Work out the finished part from the listing and answer in its coordinate system (mm). Face numbers are marked on the shaded views. A direction names the side the tool comes from. Round coordinates to 2 decimals unless told otherwise and drop trailing zeros. Write each loop counter-clockwise with the first axis right and the second up, starting at its lowest first coordinate (ties: lowest second). Pieces come first, ordered by that corner, then holes. Notation, with made-up numbers: M 7,13 L 58,13 A18 ccw 58,39 Z; hole C 4,82 d4. An arc over 180 degrees is marked long. Answer in a Markdown table with one row per item.
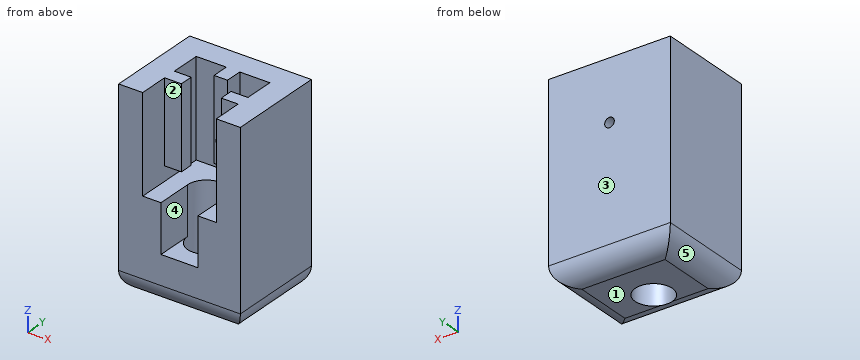
```python
from build123d import *

# Parameters (mm, degrees)
RESSALTO_EXTRUS_O1_DEPTH   = 20
ESBO_O2_W                  = 25.3
ESBO_O2_H                  = 20.3
ESBO_O2_R                  = 3.85
RESSALTO_EXTRUS_O2_DEPTH   = 20
CORTE_EXTRUS_O1_DEPTH      = 10
ESBO_O3_W                  = 3.5
ESBO_O3_H                  = 2.8
ESBO_O3_W_2                = 2.8
ESBO_O3_H_2                = 3.5
RESSALTO_EXTRUS_O3_DEPTH   = 17
CORTE_EXTRUS_O2_DEPTH      = 29.180001774
CORTE_EXTRUS_O2_DEPTH_BACK = 29.180001774
ESBO_O4_R                  = 1
FILETE1_R                  = 4


with BuildPart() as part:
    # Esboço1 → Ressalto-extrusão1 (new body)
    with BuildSketch(Plane.XY):
        Polygon((-7.65, 0), (-12.65, 0), (-12.65, 20.3), (12.65, 20.3), (12.65, 0), (7.65, 0), (7.65, 15.3), (-7.65, 15.3), align=None)
    extrude(amount=RESSALTO_EXTRUS_O1_DEPTH)

    # Esboço2 → Ressalto-extrusão2 (add)
    with BuildSketch(Plane(origin=(0, 0, 0), x_dir=(-1, 0, 0), z_dir=(0, 0, -1))):
        with Locations((0, 10.15)):
            Rectangle(ESBO_O2_W, ESBO_O2_H)
        with Locations((0, 7.65)):
            Circle(ESBO_O2_R, mode=Mode.SUBTRACT)
    extrude(amount=RESSALTO_EXTRUS_O2_DEPTH)

    # Esboço2<3> → Corte-extrusão1 (cut)
    with BuildSketch(Plane(origin=(0, 0, 0), x_dir=(-1, 0, 0), z_dir=(0, 0, -1))):
        with BuildLine():
            Line((3.85, 3.8), (2.722361108, 4.927638892))
            ThreePointArc((2.722361108, 4.927638892), (-1.473331215, 4.0930638), (-3.85, 7.65))
            Line((-3.85, 7.65), (-3.85, 0))
            Line((-3.85, 0), (3.85, 0))
            Line((3.85, 0), (3.85, 3.8))
        make_face()
        with BuildLine():
            ThreePointArc((3.85, 7.65), (3.5569362, 6.176668785), (2.722361108, 4.927638892))
            Line((2.722361108, 4.927638892), (3.85, 3.8))
            Line((3.85, 3.8), (3.85, 7.65))
        make_face()
    extrude(amount=CORTE_EXTRUS_O1_DEPTH, mode=Mode.SUBTRACT)

    # Esboço3 → Ressalto-extrusão3 (add)
    with BuildSketch(Plane.XY.offset(20)):
        with Locations((5.9, 7.65)):
            Rectangle(ESBO_O3_W, ESBO_O3_H)
        with Locations((-5.9, 7.65)):
            Rectangle(ESBO_O3_W, ESBO_O3_H)
        with Locations((0, 13.55)):
            Rectangle(ESBO_O3_W_2, ESBO_O3_H_2)
    extrude(amount=-RESSALTO_EXTRUS_O3_DEPTH)

    # Esboço4 → Corte-extrusão2 (cut, two sides: drawn at the far end of the back side and taken through both)
    with BuildSketch(Plane.XZ.offset(-15.3).offset(-CORTE_EXTRUS_O2_DEPTH_BACK)):
        with Locations(Location((0, 7.5, 0), (0, 0, 270))):
            Circle(ESBO_O4_R)
    extrude(amount=CORTE_EXTRUS_O2_DEPTH + CORTE_EXTRUS_O2_DEPTH_BACK, mode=Mode.SUBTRACT)

    # Filete1
    # the kernel refuses this fillet: 4 mm, written as the material it takes off along each edge
    with BuildSketch(Plane(origin=(12.65, -10, -20), x_dir=(-1, 0, 0), z_dir=(0, 1, 0))) as filete1_piece_1:
        with BuildLine():
            CenterArc((FILETE1_R, FILETE1_R), FILETE1_R, 180, 90)
            Line((0, FILETE1_R), (0, 0))
            Line((0, 0), (FILETE1_R, 0))
        make_face()
    extrude(amount=40.3, mode=Mode.SUBTRACT)
    with BuildSketch(Plane(origin=(-22.65, 0, -20), x_dir=(0, 0, 1), z_dir=(1, 0, 0)), Plane(origin=(22.65, 20.3, -20), x_dir=(0, 0, 1), z_dir=(-1, 0, 0))) as filete1_piece_2:
        with BuildLine():
            CenterArc((FILETE1_R, -FILETE1_R), FILETE1_R, 90, 90)
            Line((0, -FILETE1_R), (0, 0))
            Line((0, 0), (FILETE1_R, 0))
        make_face()
    extrude(amount=45.3, mode=Mode.SUBTRACT)
    with BuildSketch(Plane(origin=(-12.65, 30.3, -20), x_dir=(0, 0, 1), z_dir=(0, -1, 0))) as filete1_piece_3:
        with BuildLine():
            CenterArc((FILETE1_R, -FILETE1_R), FILETE1_R, 90, 90)
            Line((0, -FILETE1_R), (0, 0))
            Line((0, 0), (FILETE1_R, 0))
        make_face()
    extrude(amount=40.3, mode=Mode.SUBTRACT)


solid = part.part
```
1. The part is cut by section B-B (z = 8). Determine the outline of the cut face in (x, y), plus the area to 3 significant figures.
Calculated:
| item | result |
|---|---|
| outline | M -12.65,0 L -7.65,0 L -7.65,6.25 L -4.15,6.25 L -4.15,9.05 L -7.65,9.05 L -7.65,15.3 L -1.4,15.3 L -1.4,11.8 L -0.87,11.8 L -0.87,20.3 L -12.65,20.3 Z; M 0.87,11.8 L 1.4,11.8 L 1.4,15.3 L 7.65,15.3 L 7.65,9.05 L 4.15,9.05 L 4.15,6.25 L 7.65,6.25 L 7.65,0 L 12.65,0 L 12.65,20.3 L 0.87,20.3 Z |
| area | 294 mm² |
2. A tool of negligible diameter and unlimited length cuts with its end or side. For the marked faces 1 and 2, from which of +Z, -Z, +X, -X, +Y, -Y can it reach the whole face along a straight path? Write none if from no direction.
Calculated:
| item | result |
|---|---|
| face 1 | -Z, +X, -X, +Y, -Y |
| face 2 | +Z, -Y |
3. The part is cut by section A-A (x = 7). Determine the outline of the cut face in (y, z), plus the area to 3 significant figures.
Calculated:
| item | result |
|---|---|
| outline | M 0,-16 A4 ccw 4,-20 L 16.3,-20 A4 ccw 20.3,-16 L 20.3,20 L 15.3,20 L 15.3,0 L 0,0 Z; M 6.25,3 L 9.05,3 L 9.05,20 L 6.25,20 Z |
| area | 547 mm² |
4. The part is cut by section C-C (y = 4.5). Determine the outline of the cut face in (x, z), plus the area to 3 significant figures.
Calculated:
| item | result |
|---|---|
| outline | M -12.65,-16 A4 ccw -8.65,-20 L -2.21,-20 L -2.21,-10 L -3.85,-10 L -3.85,0 L -7.65,0 L -7.65,20 L -12.65,20 Z; M 2.21,-20 L 8.65,-20 A4 ccw 12.65,-16 L 12.65,20 L 7.65,20 L 7.65,0 L 3.85,0 L 3.85,-10 L 2.21,-10 Z |
| area | 578 mm² |
5. Determine the mould class of the marked faces 3, 4 and 5 for opening direction X: released by +X, released by -X, zero draft, split by the parting line, or undercut.
Calculated:
| item | result |
|---|---|
| face 3 | zero draft |
| face 4 | undercut |
| face 5 | released by -X |
6. Given pin 1 (1.8 mm diameter, centred on x = 0, z = 7.5, fed in from +Y); pin 2 (2 mm diameter, centred on x = 0, z = 15.5, fed in from -Y); pin 3 (1 mm diameter, centred on x = -6.5, z = 12, fed in from -Y); pin 4 (2 mm diameter, centred on x = -4, y = 17.5, fed in from -Z) (3 decimals), each flat-ended and moving along its own axis, determine where each tip first touches the part or whether it passes through.
Calculated:
| item | result |
|---|---|
| pin 1 | passes through |
| pin 2 | stops at y = 11.8 |
| pin 3 | stops at y = 6.25 |
| pin 4 | stops at z = -19.995 |
7. The part is cut by section D-D (z = 17). Determine the outline of the cut face in (x, y), plus the area to 3 significant figures.
Calculated:
| item | result |
|---|---|
| outline | M -12.65,0 L -7.65,0 L -7.65,6.25 L -4.15,6.25 L -4.15,9.05 L -7.65,9.05 L -7.65,15.3 L -1.4,15.3 L -1.4,11.8 L 1.4,11.8 L 1.4,15.3 L 7.65,15.3 L 7.65,9.05 L 4.15,9.05 L 4.15,6.25 L 7.65,6.25 L 7.65,0 L 12.65,0 L 12.65,20.3 L -12.65,20.3 Z |
| area | 309 mm² |
8. Consider line 1 along Z through (x, y) = (0, 14.5); line 2 along Y through (x, z) = (5.5, 14); line 3 along X through (y, z) = (15.25, 7.5). Determine where each line is inside the solid, lowest interval first. Write a range as from..to.
Calculated:
| item | result |
|---|---|
| line 1 | z = -20..0, 3..6.5, 8.5..20 |
| line 2 | y = 6.25..9.05, 15.3..20.3 |
| line 3 | x = -12.65..-7.65, -1.4..-1, 1..1.4, 7.65..12.65 |
